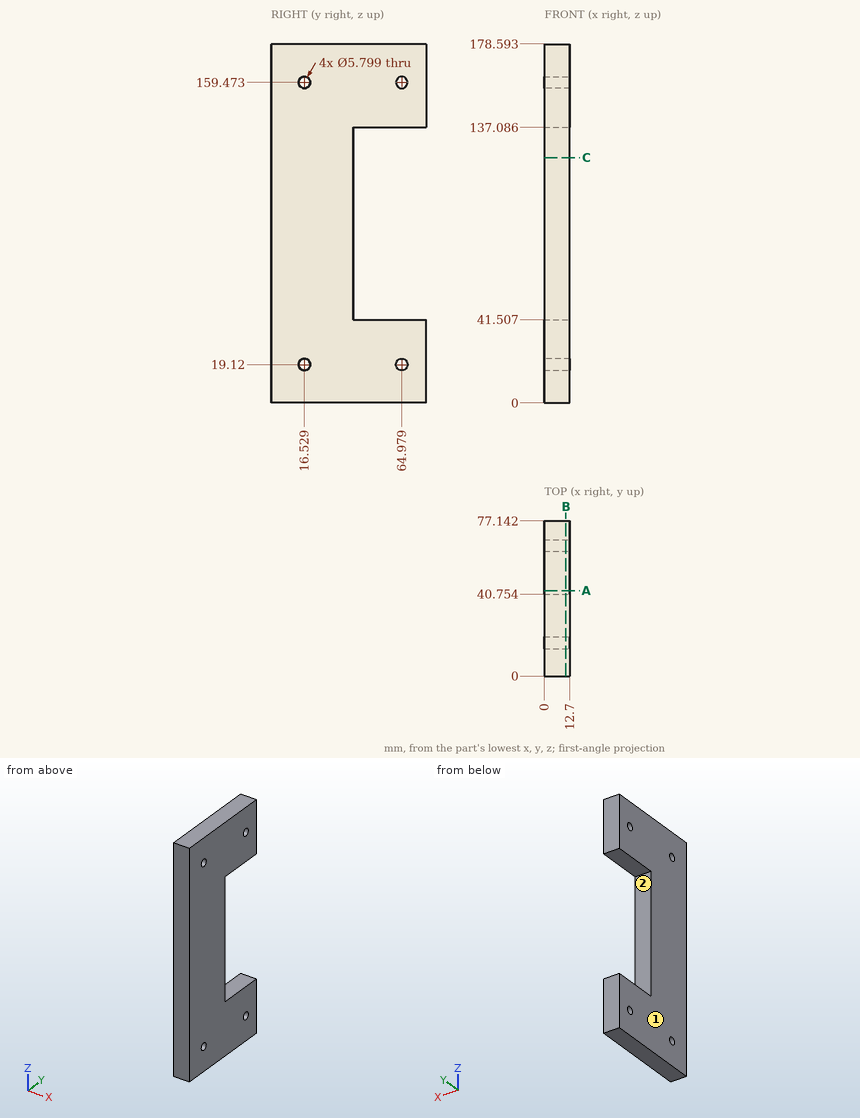
Input: dimensioned drawing with shaded views. Units: mm. Origin: part minimum x, y, z. Round coordinates to 2 decimals unless told otherwise and drop trailing zeros. Loops run counter-clockwise (first coordinate to the right, second up) from the corner with the lowest first, then second, coordinate; pieces in that order, holes last. Notation, with made-up numbers: M 85,31 L 137,31 A34 ccw 137,65 Z; hole C -15.75,34.5 d2. An arc over 180 degrees is marked long. Answer in a Markdown table with one row per item. Add a question column.
1. Section A-A (y = 42.5). Output: boundary loops of the cut face in (x, z) (1 decimal).
2. Section C-C (z = 122). Output: boundary loops of the cut face in (x, y) (1 decimal).
3. Mould query, pull axis Z, two halves, no side actions, for the marked faces 1 and 2. Classes: released by +Z, released by -Z, zero draft, split by the parting line, or undercut.
4. Ray query, probe 1 along Y at (x, z) = (0.75, 159); probe 2 along Z at (x, y) = (9, 63) (1 decimal); probe 3 along Z at (x, y) = (7.5, 60) (1 decimal). Return the intervals inside material, ascending.
5. Contact query for a flat-ended pin moving along its axis: pin 1 (3 mm diameter, centred on x = 5.5, z = 64, fed in from +Y). Output: stop coordinate, or through.
6. Section B-B (x = 10.75). Output: boundary loops of the cut face in (y, z) (1 decimal).
Values follow:
| question | item | result |
|---|---|---|
| 1 | outline | M 0,0 L 12.7,0 L 12.7,41.5 L 0,41.5 Z; M 0,137.1 L 12.7,137.1 L 12.7,178.6 L 0,178.6 Z |
| 2 | outline | M 0,0 L 12.7,0 L 12.7,40.8 L 0,40.8 Z |
| 3 | face 1 | zero draft |
| 3 | face 2 | undercut |
| 4 | probe 1 | 0 to 13.67, 19.39 to 62.12, 67.84 to 77.14 |
| 4 | probe 2 | 0 to 17, 21.2 to 41.5, 137.1 to 157.4, 161.6 to 178.6 |
| 4 | probe 3 | 0 to 41.5, 137.1 to 178.6 |
| 5 | pin 1 | y = 40.75 |
| 6 | outline | M 0,0 L 77.1,0 L 77.1,41.5 L 40.8,41.5 L 40.8,137.1 L 77.1,137.1 L 77.1,178.6 L 0,178.6 Z; hole C 16.5,19.1 d5.8; hole C 16.5,159.5 d5.8; hole C 65,19.1 d5.8; hole C 65,159.5 d5.8 |
